from build123d import *

# Parameters (mm, degrees)
SKETCH1_R           = 1.5
BOSS_EXTRUDE1_DEPTH = 4
FILLET1_R           = 1


with BuildPart() as part:
    # Sketch1 → Boss-Extrude1 (new body)
    with BuildSketch(Plane(origin=(0, 0, 0), x_dir=(1, 0, 0), z_dir=(0, 1, 0))):
        with BuildLine():
            Line((3.499999994, 18.000210437), (3.500666698, 6.911553125))
            ThreePointArc((3.500666698, 6.911553125), (4.91134936, 1.791253282), (8.744863366, -1.884568587))
            Line((8.744863366, -1.884568587), (15.782241735, -5.689211238))
            ThreePointArc((15.782241735, -5.689211238), (16.402202946, -5.79906113), (16.964928847, -5.516645723))
            Line((16.964928847, -5.516645723), (18.23595273, -4.24562184))
            ThreePointArc((18.23595273, -4.24562184), (18.560376079, -4.028849089), (18.943059511, -3.952728622))
            Line((18.943059511, -3.952728622), (24, -3.952728622))
            Line((24, -3.952728622), (24, -16.952728622))
            Line((24, -16.952728622), (-1.664016467, -3.077901019))
            ThreePointArc((-1.664016467, -3.077901019), (-3.005385337, -1.791670857), (-3.498917759, -6.5e-08))
            Line((-3.498917759, -6.5e-08), (-3.499999994, 17.999789563))
            ThreePointArc((-3.499999994, 17.999789563), (-0.000210437, 21.499999994), (3.499999994, 18.000210437))
        make_face()
        with Locations(Location((0, 0, 0), (0, 0, 270))):
            Circle(SKETCH1_R, mode=Mode.SUBTRACT)
        with Locations(Location((0, 18, 0), (0, 0, 270))):
            Circle(SKETCH1_R, mode=Mode.SUBTRACT)
    extrude(amount=BOSS_EXTRUDE1_DEPTH)

    # Fillet1
    fillet1_edges = [part.edges().sort_by_distance(p)[0] for p in [
        (-3.005385337, 4, 1.791670857),
        (3.500333346, 0, -12.455881781),
        (4.91134936, 0, -1.791253282),
        (12.26355255, 0, 3.786889912),
        (16.402202946, 0, 5.79906113),
        (17.600440788, 0, 4.881133782),
        (18.560376079, 0, 4.028849089),
        (11.167991766, 4, 10.01531482),
        (21.471529755, 0, 3.952728622),
        (11.167991766, 0, 10.01531482),
        (-3.005385337, 0, 1.791670857),
        (-3.499458876, 0, -8.999894749),
        (-0.000210437, 0, -21.499999994),
        (21.471529755, 4, 3.952728622),
        (24, 2, 16.952728622),
        (18.560376079, 4, 4.028849089),
        (17.600440788, 4, 4.881133782),
        (16.402202946, 4, 5.79906113),
        (12.26355255, 4, 3.786889912),
        (4.91134936, 4, -1.791253282),
        (3.500333346, 4, -12.455881781),
        (-0.000210437, 4, -21.499999994),
        (-3.499458876, 4, -8.999894749),
    ]]
    fillet(fillet1_edges, radius=FILLET1_R)


solid = part.part
Here's how the part is built. I have some questions about the finished solid (model axes, mm). A direction names the side the tool comes from. Coordinates: 2 decimals unless noted, no trailing zeros. Loops run counter-clockwise (first coordinate to the right, second up) from the corner with the lowest first, then second, coordinate; pieces in that order, holes last.
1. Imagine slicing it at B-B, the plane x = 0. Count the separate pieces of the cut face and the enclosed holes in it, and give its area (3 significant figures).
2. I need wall thicknesses on L1, parallel to X at y = 2.75, z = -18; L2, parallel to X at y = 0.3, z = 1; L3, parallel to X at y = 1.8, z = -14. Which ranges of each line are inside material? Lowest first, please.
3. If we mould it in two halves opening along X, with no side actions, what happens to faces 1 (the cylindrical face through (17.811, 0.301, 5.074)), 2 (the cylindrical face through (3.215, 3.699, -12.378)), 3 (the cylindrical face through (10.83, 0.3, 9.51))? For each: pulls with the +X half, pulls with the -X half, needs draft (parallel to the pull), parting line crosses it, or undercut.
4. Imagine slicing it at A-A, the plane y = 2.55. Please give me the cut outline in (x, z), and give its area (3 significant figures).
5. For faces 4 (the cylindrical face through (17.811, 3.699, 5.074)), 5 (the flat face through (17.59, 1.99, 4.89)), 6 (the cylindrical face through (21.51, 0.3, 4.24)), 7 (the cylindrical face through (21.51, 3.7, 4.24)), which set-ups out of +Z, -Z, +X, -X, +Y, -Y let a thin tool reach every point of the face, with its end or its side?
6. For P1, Ø2, axis at y = 0.5, z = -7.5, coming from the +X side; P2, Ø4, axis at x = 3.5, z = 9, coming from the -Y side; P3, Ø1.5, axis at x = 3, y = 3, coming from the -Z side; P4, Ø2, axis at x = 11.5, y = 1, coming from the +Z side, each with a flat end and sliding along its axis, tell me the tip position at first contact or that it passes through.
Taken from the geometry:
1. separate pieces: 3
1. enclosed holes: 0
1. area: 77.0 mm2
2. L1: x = -3.5 to -1.5, 1.5 to 3.5
2. L2: x = -3.05 to -1.12, 1.12 to 6.93
2. L3: x = -3.5 to 3.5
3. face 1: undercut
3. face 2: pulls with the +X half
3. face 3: pulls with the -X half
4. outline: (-3.5, -18) arc R3.5 ccw to (3.5, -18) - (3.5, -6.91) arc R10 cw to (8.74, 1.88) - (15.78, 5.69) arc R1 cw to (16.96, 5.52) - (18.24, 4.25) arc R1 ccw to (18.94, 3.95) - (24, 3.95) - (24, 15.28) arc R1 ccw to (22.52, 16.15) - (-1.66, 3.08) arc R3.5 ccw to (-3.5, 0) - close; hole circle Ø3 at (0, -18); hole circle Ø3 at (0, 0)
4. area: 332 mm2
5. face 4: -Z, +Y
5. face 5: -Z, +Y, -Y
5. face 6: -Z, +X, -Y
5. face 7: -Z, +X, +Y
6. P1: stops at x = 3.5
6. P2: passes through
6. P3: stops at z = -20.68
6. P4: stops at z = 10.74
